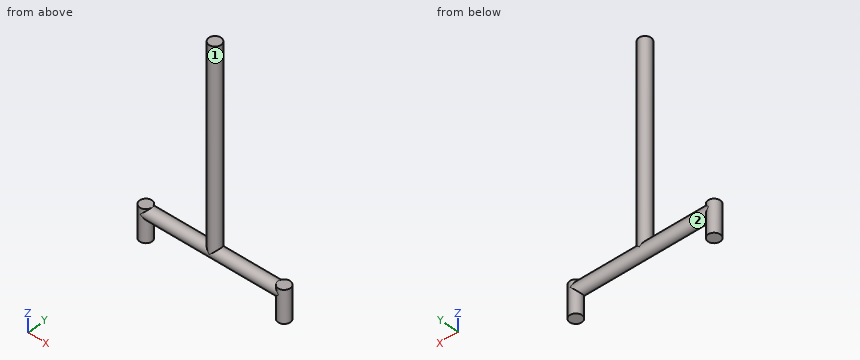
Autodesk Fusion 360 part; units mm, degrees
sketch "Sketch1" plane through (0, 0, 0) normal (0, 0, 1) x (1, 0, 0)
  circle A0 centre (-180, 0) radius 8
  circle A1 centre (0, 0) radius 8
  dimension "d1" = 16
  dimension "d2" = 16
  dimension "d3" = 180
extrude "Extrude1" add sketch "Sketch1" along normal blind 42 makes body 1 at (-172.0099, -0.3988, 28) makes body 2 at (7.9901, -0.3988, 28)
sketch "Sketch2" plane through (0, 0, 0) normal (1, 0, 0) x (0, 1, 0)
  line L0 (8, 42) -> (-8, 42)
  line L1 (8, 0) -> (-8, 0)
  line L2 (0, 42) -> (0, 34) construction
  circle A0 centre (0, 34) radius 8
  dimension "d6" = 8
extrude "Extrude2" add sketch "Sketch2" against normal blind 180 bodies 1 2
ref_plane "WorkPlane1" through (-100.4607, 0, 42) normal (0, 0, 1) x (0, -1, 0)
sketch "Sketch3" plane through (-100.4607, 0, 42) normal (0, 0, 1) x (1, 0, 0)
  arc A0 (-71.5393, 0) -> (-79.5393, 8) centre (-79.5393, 0) ccw
  arc A1 (-79.5393, -8) -> (-71.5393, 0) centre (-79.5393, 0) ccw
  arc A2 (-79.5393, -8) -> (-79.5393, 8) centre (-79.5393, 0) ccw
  arc A3 (100.4607, 8) -> (100.4607, -8) centre (100.4607, 0) ccw
  arc A4 (92.4607, 0) -> (100.4607, -8) centre (100.4607, 0) ccw
  arc A5 (100.4607, 8) -> (92.4607, 0) centre (100.4607, 0) ccw
  circle A6 centre (100.4607, 0) radius 8
  circle A7 centre (-79.5393, 0) radius 8
  line L0 (-79.5393, 0) -> (10.4607, 0) construction
  circle A8 centre (10.4607, 0) radius 8
  dimension "d10" = 90
  dimension "d11" = 16
extrude "Extrude3" add sketch "Sketch3" against normal blind 8 contours A8 bodies 1
extrude "Extrude4" add 1 faces at (-92.292, 0.3187, 42) along direction (0, 0, 1) blind 250 on bodies 1 bodies 1
Here's how the part is built. I have some questions about the finished solid (model axes, mm). Face numbers are marked on the shaded views. Round coordinates to 2 decimals unless told otherwise and drop trailing zeros. Write each loop counter-clockwise with the first axis right and the second up, starting at its lowest first coordinate (ties: lowest second). Pieces come first, ordered by that corner, then holes.
1. Suppose I cut it at B-B (y = -4). List the corners of the cut face in (x, z) for me.
2. If we mould it in two halves opening along Z, with no side actions, what happens to the marked faces 1 and 2? For each: released by +Z, released by -Z, zero draft, split by the parting line, or undercut.
3. Suppose I cut it at A-A (z = 37.5). List the corners of the cut face in (x, y) for me, and give its area (3 significant figures).
4. I need wall thicknesses on L1, parallel to Z at x = -28, y = 0.75; L2, parallel to Y at x = -32, z = 33; L3, parallel to Z at x = -106.5, y = 6. Which ranges of each line are inside material? Lowest first, please.
5. Suppose I cut it at C-C (x = -145). List the corners of the cut face in (y, z) for me, and give its area (3 significant figures).
6. Suppose I cut it at D-D (z = 123). List the corners of the cut face in (x, y) for me.
7. Will these pins go through, and if not, where does the flat tip stop? pin 1 Ø3 at (y, z) = (-4, 201.5) entering from -X; pin 2 Ø8 at (y, z) = (2, 248) entering from +X; pin 3 Ø8 at (x, y) = (-176.5, 2) entering from +Z; pin 4 Ø6 at (x, z) = (-88.5, 38) entering from +Y.
Answer sheet:
1. outline: (-186.93, 0) - (-173.07, 0) - (-173.07, 27.07) - (-6.93, 27.07) - (-6.93, 0) - (6.93, 0) - (6.93, 42) - (-6.93, 42) - (-6.93, 40.93) - (-83.07, 40.93) - (-83.07, 292) - (-96.93, 292) - (-96.93, 40.93) - (-173.07, 40.93) - (-173.07, 42) - (-186.93, 42) - close
2. face 1: zero draft
2. face 2: split by the parting line
3. outline: (-176.5, -7.19) - (-93.5, -7.19) arc R8 ccw to (-86.5, -7.19) - (-3.5, -7.19) arc R8 ccw (long way) to (-3.5, 7.19) - (-86.5, 7.19) arc R8 ccw to (-93.5, 7.19) - (-176.5, 7.19) arc R8 ccw (long way) to start
3. area: 2,810 mm2
4. L1: z = 26.04 to 41.96
4. L2: y = -7.94 to 7.94
4. L3: z = 28.71 to 39.29
5. outline: circle Ø16 at (0, 34)
5. area: 201 mm2
6. outline: circle Ø16 at (-90, 0)
7. pin 1: stops at x = -97.6
7. pin 2: stops at x = -82
7. pin 3: stops at z = 42
7. pin 4: stops at y = 8
